Geometry check sheet. Reference: the model listing, model coordinates, mm. Face numbers are marked on the shaded views. A direction names the side the tool comes from. Give positions to 0.01 mm unless a question says otherwise; leave off trailing zeros. Order: outer loops, then holes, each group sorted by start corner. A loop starts at its lowest first (then second) coordinate and runs counter-clockwise, first axis right, second up. Notation, with made-up numbers: (10, -38.5) - (52, -38.5) arc R17 ccw to (52, -34.5) - close; hole circle Ø4 at (-7, 78.25). An arc over 180 degrees is marked (long way). Put each result on its own line as item: value. Start each with the question number.
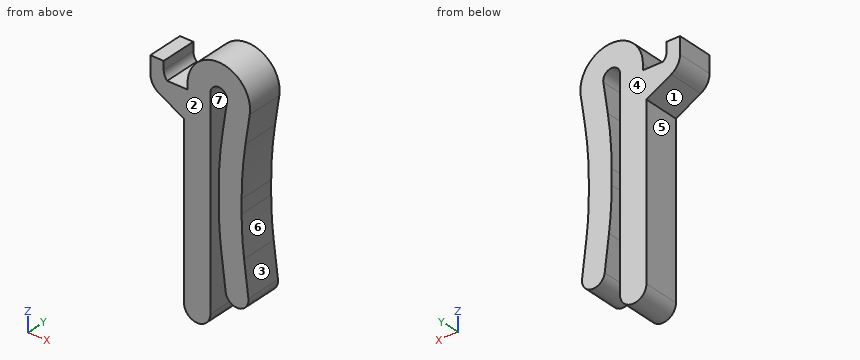
```python
from build123d import *

# Parameters (mm, degrees)
F1_DEPTH = 3.302


with BuildPart() as f1:
    # F0 (on Front) → F1 (new body)
    with BuildSketch(Plane.XZ):
        with BuildLine():
            Line((-1.1938, 18.9738), (-2.7178, 18.9738))
            ThreePointArc((-2.7178, 18.9738), (-2.95275, 19.32305), (-3.0353, 19.7358))
            Line((-3.0353, 19.7358), (-3.0353, 20.4978))
            Line((-3.0353, 20.4978), (-4.2418, 20.4978))
            Line((-4.2418, 20.4978), (-4.2418, 18.9738))
            ThreePointArc((-4.2418, 18.9738), (-4.027637, 18.19849), (-3.445879, 17.643037))
            Line((-3.445879, 17.643037), (-1.1938, 16.4338))
            Line((-1.1938, 16.4338), (-1.1938, 1.1938))
            ThreePointArc((-1.1938, 1.1938), (0, 0), (1.1938, 1.1938))
            Line((1.1938, 1.1938), (1.1938, 19.5072))
            ThreePointArc((1.1938, 19.5072), (2.011944, 20.267129), (2.709527, 19.395217))
            Line((2.709527, 19.395217), (2.300525, 16.642347))
            ThreePointArc((2.300525, 16.642347), (2.042099, 14.315723), (1.9558, 11.976382))
            Line((1.9558, 11.976382), (1.9558, 10.582195))
            ThreePointArc((1.9558, 10.582195), (2.016106, 8.626227), (2.196796, 6.67769))
            Line((2.196796, 6.67769), (2.58224, 3.567194))
            ThreePointArc((2.58224, 3.567194), (3.73672, 2.667287), (4.636627, 3.821767))
            Line((4.636627, 3.821767), (4.251183, 6.932264))
            ThreePointArc((4.251183, 6.932264), (4.082274, 8.753757), (4.0259, 10.582195))
            Line((4.0259, 10.582195), (4.0259, 11.823441))
            ThreePointArc((4.0259, 11.823441), (4.112199, 14.162782), (4.370625, 16.489406))
            Line((4.370625, 16.489406), (4.75715, 19.090996))
            ThreePointArc((4.75715, 19.090996), (2.164469, 22.331602), (-0.8763, 19.5072))
            Line((-0.8763, 19.5072), (-0.8763, 18.9738))
            Line((-0.8763, 18.9738), (-1.1938, 18.9738))
        make_face()
    extrude(amount=F1_DEPTH)


solid = f1.part
```
Item 1: Cross-section at D-D (x = 0). Enter the section's corners in (y, z), and give its area (3 significant figures).
Item 2: Cross-section at A-A (z = 8.25). Enter the section's corners in (x, y), and give its area (3 significant figures).
Item 3: Set-up check for the marked faces 4, 5, 6 and 7: record each of +Z, -Z, +X, -X, +Y, -Y from which the full face is reachable in a straight line by a thin tool's end or side.
Item 4: Cross-section at C-C (z = 20). Enter the section's corners in (x, y), and give its area (3 significant figures).
Item 5: Thickness scan on line 1 along X through (y, z) = (-2.9, 16.5); line 2 along X through (y, z) = (-0.3, 10); line 3 along Z through (x, y) = (3, -1.7). Record the ranges inside material, lowest first.
Item 6: Cross-section at B-B (y = -3). Enter the section's corners in (x, z).
Item 7: Release check for a two-part mould opening along Z. For the marked faces 1, 2 and 3 record: +Z half, -Z half, draft (parallel to the pull), parting line (faces both ways), or undercut.
Item 8: Gauge pin test, flat ends, axial feed: pin 1 Ø1.3 at (x, y) = (-4, -1) entering from +Z; pin 2 Ø1.4 at (y, z) = (-2.5, 11) entering from +X; pin 3 Ø1.7 at (y, z) = (-2, 10.5) entering from -X. Record the tip position at first contact, or that the pin passes through.
Recorded:
1. outline: (-3.3, 0) - (0, 0) - (0, 21.56) - (-3.3, 21.56) - close
1. area: 71.2 mm^2
2. outline: (-1.19, -3.3) - (1.19, -3.3) - (1.19, 0) - (-1.19, 0) - close; (2.04, -3.3) - (4.12, -3.3) - (4.12, 0) - (2.04, 0) - close
2. area: 14.7 mm^2
3. face 4: +Z, -Z, +X, -X, +Y
3. face 5: -Z, -X, +Y, -Y
3. face 6: +X, +Y, -Y
3. face 7: -Z, +Y, -Y
4. outline: (-4.24, -3.3) - (-3.04, -3.3) - (-3.04, 0) - (-4.24, 0) - close; (-0.83, -3.3) - (1.37, -3.3) - (1.37, 0) - (-0.83, 0) - close; (2.54, -3.3) - (4.74, -3.3) - (4.74, 0) - (2.54, 0) - close
4. area: 18.6 mm^2
5. line 1: x = -1.32 to 1.19, 2.28 to 4.37
5. line 2: x = -1.19 to 1.19, 1.96 to 4.03
5. line 3: z = 2.86 to 22.14
6. outline: (-4.24, 18.97) arc R1.51 ccw to (-3.45, 17.64) - (-1.19, 16.43) - (-1.19, 1.19) arc R1.19 ccw to (1.19, 1.19) - (1.19, 19.51) arc R0.76 cw (long way) to (2.71, 19.4) - (2.3, 16.64) arc R31.75 ccw to (1.96, 11.98) - (1.96, 10.58) arc R31.75 ccw to (2.2, 6.68) - (2.58, 3.57) arc R1.04 ccw to (4.64, 3.82) - (4.25, 6.93) arc R29.68 cw to (4.03, 10.58) - (4.03, 11.82) arc R31.75 cw to (4.37, 16.49) - (4.76, 19.09) arc R2.83 ccw (long way) to (-0.88, 19.51) - (-0.88, 18.97) - (-2.72, 18.97) arc R1.07 cw to (-3.04, 19.74) - (-3.04, 20.5) - (-4.24, 20.5) - close
7. face 1: -Z half
7. face 2: draft
7. face 3: undercut
8. pin 1: stops at z = 20.5
8. pin 2: stops at x = 4.03
8. pin 3: stops at x = -1.19
